from build123d import *

# Parameters (mm, degrees)
SKETCH_4_W          = 20.69495493
SKETCH_4_H          = 9.945675455
EXTRUDE_4_DEPTH     = 30
CHAMFER_1_SIZE      = 20.5
CHAMFER_2_SIZE      = 3
SKETCH_5_R          = 2.499998555
CUT_EXTRUDE_1_DEPTH = 43.013443482


with BuildPart() as part:
    # Эскиз4 → Вытянуть4 (new body)
    with BuildSketch(Plane(origin=(0, 0, 0), x_dir=(1, 0, 0), z_dir=(0, 1, 0))):
        with Locations((17.333074787, 12.950285074)):
            Rectangle(SKETCH_4_W, SKETCH_4_H)
    extrude(amount=EXTRUDE_4_DEPTH)

    # Фаска1
    chamfer_1_edges = [part.edges().sort_by_distance(p)[0] for p in [
        (27.680552252, 30, -12.950285073),
    ]]
    chamfer(chamfer_1_edges, length=CHAMFER_1_SIZE)

    # Фаска2
    chamfer_2_edges = [part.edges().sort_by_distance(p)[0] for p in [
        (27.680552252, 0, -12.950285073),
    ]]
    chamfer(chamfer_2_edges, length=CHAMFER_2_SIZE)

    # Эскиз5 → Вырез-Вытянуть1 (cut, through all)
    with BuildSketch(Plane.XY.offset(-7.977447346)):
        with Locations((18.250594968, 8.095401179)):
            Circle(SKETCH_5_R)
    extrude(amount=-CUT_EXTRUDE_1_DEPTH, mode=Mode.SUBTRACT)


solid = part.part
Work out the finished part from the listing and answer in its coordinate system (mm). Give positions to 0.01 mm unless a question says otherwise; leave off trailing zeros. Write each loop counter-clockwise with the first axis right and the second up, starting at its lowest first coordinate (ties: lowest second). Pieces come first, ordered by that corner, then holes.
Q1. The part is cut by section D-D on y = 22.5. Give the vertices of the cut face in (x, z).
Answer:
outline: (6.99, -17.92) - (14.68, -17.92) - (14.68, -7.98) - (6.99, -7.98) - close
Q2. The part is cut by section C-C on x = 12.5. Give the vertices of the cut face in (y, z).
Answer:
outline: (0, -17.92) - (24.68, -17.92) - (24.68, -7.98) - (0, -7.98) - close
Q3. The part is cut by section A-A on z = -11.25. Give the vertices of the cut face in (x, y).
Answer:
outline: (6.99, 0) - (24.68, 0) - (27.68, 3) - (27.68, 9.5) - (7.18, 30) - (6.99, 30) - close; hole circle Ø5 at (18.25, 8.1)
Q4. Straight lines are drawn through the part: L1, parallel to Y at x = 9.5, z = -9.5; L2, parallel to X at y = 9.5, z = -14.25; L3, parallel to Y at x = 19.25, z = -12.25. For each, find the intervals that lie inside material, in ascending order.
Answer:
L1: y = 0 to 27.68
L2: x = 6.99 to 16.18, 20.32 to 27.68
L3: y = 0 to 5.8, 10.39 to 17.93
Q5. For a pull along X with two mould halves and no side action, classify faces 1 (the face through (17.29, 19.89, -12.88)), 2 (the face through (15.753, 8.205, -12.881)), 3 (the face through (6.986, 15, -13)) as released by +X, released by -X, zero draft, split by the parting line, or undercut.
Answer:
face 1: released by +X
face 2: undercut
face 3: released by -X
Q6. The part is cut by section B-B on x = 17.25. Give the vertices of the cut face in (y, z), and give its area (3 significant figures).
Answer:
outline: (0, -17.92) - (5.8, -17.92) - (5.8, -7.98) - (0, -7.98) - close; (10.39, -17.92) - (19.93, -17.92) - (19.93, -7.98) - (10.39, -7.98) - close
area: 153 mm2
Q7. Given pin 1 (3 mm diameter, centred on x = 18.25, y = 8.1, fed in from -Z); pin 2 (1.5 mm diameter, centred on x = 15, z = -10.5, fed in from +Y), each flat-ended and moving along its own axis, determine where each tip first touches the part or whether it passes through.
Answer:
pin 1: passes through
pin 2: stops at y = 22.93
